For this review, take the finished solid that the model builds, in its own axes (mm). A direction names the side the tool comes from. Give positions to 0.01 mm unless a question says otherwise; leave off trailing zeros. Order: outer loops, then holes, each group sorted by start corner. A loop starts at its lowest first (then second) coordinate and runs counter-clockwise, first axis right, second up.
from build123d import *

# Parameters (mm, degrees)
BOSS_EXTRUDE1_DEPTH = 2.44
BOSS_EXTRUDE2_DEPTH = 1
BOSS_EXTRUDE3_START = 1
BOSS_EXTRUDE3_DEPTH = 1
SKETCH4_W           = 8.3
SKETCH4_H           = 1.59
CUT_EXTRUDE1_DEPTH  = 10
FILLET1_R           = 0.5
SKETCH5_R           = 0.15
CUT_EXTRUDE2_DEPTH  = 0.5
SKETCH6_W           = 2.05
SKETCH6_H           = 2.05
CUT_EXTRUDE3_DEPTH  = 0.5


with BuildPart() as part:
    # Sketch1 → Boss-Extrude1 (new body)
    with BuildSketch(Plane(origin=(0, 0, 0), x_dir=(1, 0, 0), z_dir=(0, 1, 0))):
        with BuildLine():
            Line((5, 6.154307787), (5, 4.25))
            Line((5, 4.25), (-5, 4.25))
            Line((-5, 4.25), (-5, -4.25))
            Line((-5, -4.25), (5, -4.25))
            Line((5, -4.25), (5, -6.154307787))
            ThreePointArc((5, -6.154307787), (11.154307787, 0), (5, 6.154307787))
        make_face()
    extrude(amount=BOSS_EXTRUDE1_DEPTH)

    # Sketch2 → Boss-Extrude2 (add)
    with BuildSketch(Plane(origin=(0, 2.44, 0), x_dir=(1, 0, 0), z_dir=(0, 1, 0))):
        with BuildLine():
            Line((5, 6.154307787), (5, -6.154307787))
            ThreePointArc((5, -6.154307787), (11.154307787, 0), (5, 6.154307787))
        make_face()
    extrude(amount=BOSS_EXTRUDE2_DEPTH)

    # Sketch3 → Boss-Extrude3 (add)
    with BuildSketch(Plane.XZ.offset(BOSS_EXTRUDE3_START)):
        with BuildLine():
            Line((5, 6.154307787), (5, -6.154307787))
            ThreePointArc((5, -6.154307787), (11.154307787, 0), (5, 6.154307787))
        make_face()
    extrude(amount=-BOSS_EXTRUDE3_DEPTH)

    # Sketch4 → Cut-Extrude1 (cut)
    with BuildSketch(Plane.ZY.offset(5)):
        with Locations((0, 1.545)):
            Rectangle(SKETCH4_W, SKETCH4_H)
    extrude(amount=-CUT_EXTRUDE1_DEPTH, mode=Mode.SUBTRACT)

    # Fillet1
    fillet1_edges = [part.edges().sort_by_distance(p)[0] for p in [
        (5, 1.22, -6.154307787),
        (5, 1.22, 6.154307787),
        (11.154307787, 3.44, 0),
        (5, 3.44, 0),
        (11.154307787, -1, 0),
        (5, -1, 0),
    ]]
    fillet(fillet1_edges, radius=FILLET1_R)

    # Sketch5 → Cut-Extrude2 (cut)
    with BuildSketch(Plane(origin=(0, 3.44, 0), x_dir=(1, 0, 0), z_dir=(0, 1, 0))):
        with Locations(Location((9.172175781, 1.326041416, 0), (0, 0, 270))):
            Circle(SKETCH5_R)
        with Locations(Location((8.125504079, 0.698038394, 0), (0, 0, 270))):
            Circle(SKETCH5_R)
        with Locations(Location((9.439658549, 0, 0), (0, 0, 270))):
            Circle(SKETCH5_R)
        with Locations(Location((9.172175781, -1.326041416, 0), (0, 0, 90))):
            Circle(SKETCH5_R)
        with Locations(Location((8.125504079, -0.698038394, 0), (0, 0, 90))):
            Circle(SKETCH5_R)
    extrude(amount=-CUT_EXTRUDE2_DEPTH, mode=Mode.SUBTRACT)

    # Sketch6 → Cut-Extrude3 (cut)
    with BuildSketch(Plane(origin=(0, 2.44, 0), x_dir=(1, 0, 0), z_dir=(0, 1, 0))):
        with Locations((0, -2.225)):
            Rectangle(SKETCH6_W, SKETCH6_H)
        with Locations((0, 2.225)):
            Rectangle(SKETCH6_W, SKETCH6_H)
    extrude(amount=-CUT_EXTRUDE3_DEPTH, mode=Mode.SUBTRACT)


solid = part.part
1) We need section A-A on x = -2. Give the boundary of the cut face in (y, z), then the cut area to 3 significant figures.
Answer sheet:
outline: (0, -4.25) - (2.44, -4.25) - (2.44, 4.25) - (0, 4.25) - close; hole (0.75, -4.15) - (2.34, -4.15) - (2.34, 4.15) - (0.75, 4.15) - close
area: 7.54 mm2
2) We need section D-D on y = 1.3. Give the boundary of the cut face in (x, z).
Answer sheet:
outline: (-5, -4.25) - (5, -4.25) - (5, -5.63) arc R0.5 ccw to (5.54, -6.13) arc R6.15 ccw to (5.54, 6.13) arc R0.5 ccw to (5, 5.63) - (5, 4.25) - (-5, 4.25) - (-5, 4.15) - (5, 4.15) - (5, -4.15) - (-5, -4.15) - close
3) Clearance check with flat-ended pins moving along their axes: pin 1 (4 mm diameter, centred on x = -1.5, z = 0, fed in from +Y); pin 2 (2.5 mm diameter, centred on x = 0, y = 1.5, fed in from -Z); pin 3 (2.5 mm diameter, centred on x = -1, y = 2, fed in from +Z). State where each tip first meets the part, or that it passes through.
Answer sheet:
pin 1: stops at y = 2.44
pin 2: stops at z = -4.25
pin 3: stops at z = 4.25
4) Draft analysis for pull direction Z (two halves, no side actions). For faces 1 (the face through (0, 0.75, 0)), 2 (the face through (5, -0.3, 0.1)), 3 (the face through (11.153, 1.196, -0.128)), 4 (the face through (5, 2, 0)), state which applies: +Z half, -Z half, draft (parallel to the pull), parting line (faces both ways), or undercut.
Answer sheet:
face 1: undercut
face 2: draft
face 3: parting line
face 4: undercut
5) We need section B-B on y = 0.45. Give the boundary of the cut face in (x, z), then the cut area to 3 significant figures.
Answer sheet:
outline: (-5, -4.25) - (5, -4.25) - (5, -5.63) arc R0.5 ccw to (5.54, -6.13) arc R6.15 ccw to (5.54, 6.13) arc R0.5 ccw to (5, 5.63) - (5, 4.25) - (-5, 4.25) - close
area: 144 mm2
6) To check wall thickness, follow line 1 (Z direction, x = -3.25, y = 0.15); line 2 (X direction, y = 2.4, z = 2.5) (3 decimals); line 3 (X direction, y = 3.35, z = 0). State the ranges of each line that lie inside material, in increasing order.
Answer sheet:
line 1: z = -4.25 to 4.25
line 2: x = -5 to -1.025, 1.025 to 10.624
line 3: x = 5.21 to 9.29, 9.59 to 10.94
7) We need section C-C on x = 0.5. Give the boundary of the cut face in (y, z).
Answer sheet:
outline: (0, -4.25) - (2.44, -4.25) - (2.44, -3.25) - (2.34, -3.25) - (2.34, -4.15) - (0.75, -4.15) - (0.75, 4.15) - (2.34, 4.15) - (2.34, 3.25) - (2.44, 3.25) - (2.44, 4.25) - (0, 4.25) - close; (2.34, -1.2) - (2.44, -1.2) - (2.44, 1.2) - (2.34, 1.2) - close
8) Tool access review of faces 5 (the face through (0, 0, 0)), 6 (the face through (-5, 0.58, -0.02)): name each direction out of +Z, -Z, +X, -X, +Y, -Y from which nothing blocks a thin tool from reaching the whole face with its end or side.
Answer sheet:
face 5: +Z, -Z, -X, -Y
face 6: +Z, -Z, -X, +Y, -Y
